from build123d import *

# Parameters (mm, degrees)
SZKIC1_W                    = 200
SZKIC1_H                    = 5
SZKIC1_W_2                  = 46
SZKIC1_H_2                  = 37
SZKIC1_W_3                  = 24
SZKIC1_W_4                  = 125
DODANIE_WYCI_GNI_CIE1_DEPTH = 5
SZKIC1_4_W                  = 125
SZKIC1_4_H                  = 5
SZKIC1_4_W_2                = 200
DODANIE_WYCI_GNI_CIE2_DEPTH = 86


with BuildPart() as part:
    # Szkic1 → Dodanie-wyci_gni_cie1 (new body)
    with BuildSketch(Plane(origin=(0, 0, 0), x_dir=(1, 0, 0), z_dir=(0, 1, 0))):
        with Locations((-8.765553919, -32.5)):
            Rectangle(SZKIC1_W, SZKIC1_H)
        with Locations((44.234446081, 91.5)):
            Rectangle(SZKIC1_W_2, SZKIC1_H_2)
        with Locations((79.234446081, 91.5)):
            Rectangle(SZKIC1_W_3, SZKIC1_H_2)
        with Locations((-46.265553919, 75.5)):
            Rectangle(SZKIC1_W_4, SZKIC1_H)
        Polygon((16.234446081, 73), (21.234446081, 73), (21.234446081, 110), (21.234446081, 115), (16.234446081, 115), (16.234446081, 78), align=None)
        Polygon((67.234446081, 110), (91.234446081, 110), (91.234446081, 115), (21.234446081, 115), (21.234446081, 110), align=None)
        with BuildLine():
            Line((91.234446081, -30), (91.234446081, 21.5))
            Line((91.234446081, 21.5), (70.234446081, 21.5))
            ThreePointArc((70.234446081, 21.5), (65.113125737, 19.378679656), (67.234446081, 24.5))
            Line((67.234446081, 24.5), (67.234446081, 73))
            Line((67.234446081, 73), (21.234446081, 73))
            Line((21.234446081, 73), (16.234446081, 73))
            Line((16.234446081, 73), (-108.765553919, 73))
            Line((-108.765553919, 73), (-108.765553919, -30))
            Line((-108.765553919, -30), (91.234446081, -30))
        make_face()
        with BuildLine():
            Line((70.234446081, 21.5), (91.234446081, 21.5))
            Line((91.234446081, 21.5), (91.234446081, 73))
            Line((91.234446081, 73), (67.234446081, 73))
            Line((67.234446081, 73), (67.234446081, 24.5))
            ThreePointArc((67.234446081, 24.5), (69.355766424, 23.621320344), (70.234446081, 21.5))
        make_face()
    extrude(amount=-DODANIE_WYCI_GNI_CIE1_DEPTH)

    # Szkic1_4 → Dodanie-wyci_gni_cie2 (add)
    with BuildSketch(Plane(origin=(0, 0, 0), x_dir=(1, 0, 0), z_dir=(0, 1, 0))):
        with Locations((-46.265553919, 75.5)):
            Rectangle(SZKIC1_4_W, SZKIC1_4_H)
        Polygon((16.234446081, 73), (21.234446081, 73), (21.234446081, 110), (21.234446081, 115), (16.234446081, 115), (16.234446081, 78), align=None)
        Polygon((67.234446081, 110), (91.234446081, 110), (91.234446081, 115), (21.234446081, 115), (21.234446081, 110), align=None)
        with Locations((-8.765553919, -32.5)):
            Rectangle(SZKIC1_4_W_2, SZKIC1_4_H)
    extrude(amount=DODANIE_WYCI_GNI_CIE2_DEPTH)


solid = part.part
For this review, take the finished solid that the model builds, in its own axes (mm). A direction names the side the tool comes from. Round coordinates to 2 decimals unless told otherwise and drop trailing zeros. Loops run counter-clockwise (first coordinate to the right, second up) from the corner with the lowest first, then second, coordinate; pieces in that order, holes last. Notation, with made-up numbers: (37, 82) - (46, 82) arc R8 cw to (46, 97) - close; hole circle Ø5 at (-34, -16). An arc over 180 degrees is marked (long way). Use one line per item in the form item = value.
Item 1: Consider section A-A on y = 61.5. Write out the cut boundary in (x, z), then the cut area to 4 significant figures.
Answers:
outline = (-108.77, -78) - (16.23, -78) - (16.23, -115) - (91.23, -115) - (91.23, -110) - (21.23, -110) - (21.23, -73) - (-108.77, -73) - close; (-108.77, 30) - (91.23, 30) - (91.23, 35) - (-108.77, 35) - close
area = 2,185 mm^2
Item 2: Tool access review of faces 1 (the flat face through (-45, 42, -73)), 2 (the flat face through (-47, 40, -78)), 3 (the flat face through (-10, 41, 35)), 4 (the flat face through (21.234, 42, -91)): name each direction out of +Z, -Z, +X, -X, +Y, -Y from which nothing blocks a thin tool from reaching the whole face with its end or side.
Answers:
face_1 = +X, -X, +Y
face_2 = -Z, -X, +Y, -Y
face_3 = +Z, +X, -X, +Y, -Y
face_4 = +X, +Y
Item 3: Consider section C-C on z = -5. Write out the cut boundary in (x, y).
Answers:
outline = (-108.77, -5) - (91.23, -5) - (91.23, 0) - (-108.77, 0) - close
Item 4: Consider section B-B on x = 61.5. Write out the cut boundary in (y, z).
Answers:
outline = (-5, -115) - (86, -115) - (86, -110) - (0, -110) - (0, 30) - (86, 30) - (86, 35) - (-5, 35) - close
Item 5: Consider section D-D on x = -0.5. Write out the cut boundary in (y, z), then the cut area to 4 significant figures.
Answers:
outline = (-5, -78) - (86, -78) - (86, -73) - (0, -73) - (0, 30) - (86, 30) - (86, 35) - (-5, 35) - close
area = 1,425 mm^2
Item 6: Clearance check with flat-ended pins moving along their axes: P1, Ø8, axis at x = 67.23, z = -21.5, coming from the +Y side; P2, Ø8, axis at y = 7.5, z = -33, coming from the +X side; P3, Ø18.5, axis at y = 40.5, z = -90.5, coming from the -X side; P4, Ø11, axis at y = 34.5, z = -89.5, coming from the +X side. State where each tip first meets the part, or that it passes through.
Answers:
P1 = 0
P2 = through
P3 = 16.23
P4 = 21.23
Item 7: For line 1 (Z direction, x = 74.5, y = 57); line 2 (Z direction, x = -56, y = 51.5); line 3 (X direction, y = -1, z = -21), list the stretches that pass through material, from the lowest coordinate up.
Answers:
line_1 = -115 to -110, 30 to 35
line_2 = -78 to -73, 30 to 35
line_3 = -108.77 to 64.28, 70.19 to 91.23
